Geometry check sheet. Reference: drawing and pictorial views, mm from the part's lowest x, y, z. A direction names the side the tool comes from. Round coordinates to 2 decimals unless told otherwise and drop trailing zeros. Order: outer loops, then holes, each group sorted by start corner. A loop starts at its lowest first (then second) coordinate and runs counter-clockwise, first axis right, second up.
(1) Set-up check for the marked faces 1, 2 and 3: record each of +Z, -Z, +X, -X, +Y, -Y from which the full face is reachable in a straight line by a thin tool's end or side.
(2) Go/stop test with flat-tipped pins: pin 1 (3 mm diameter, centred on y = 16.5, z = 2.5, fed in from +X); pin 2 (3.5 mm diameter, centred on x = 41.5, z = 7, fed in from -Y); pin 3 (3 mm diameter, centred on x = 48.5, z = 8.5, fed in from +Y). Record where each tip stops, or that it passes through.
(3) Sectioned sample at A-A (x = 54.5). Record the boundary of the cut face in (y, z).
(4) Sectioned sample at C-C (z = 7.5). Record the boundary of the cut face in (x, y).
(5) Sectioned sample at D-D (x = 38). Record the boundary of the cut face in (y, z).
(6) Sectioned sample at B-B (y = 79.5). Record the boundary of the cut face in (x, z).
(7) Release check for a two-part mould opening along X. For the marked faces 4, 5, 6 and 7 record: +X half, -X half, draft (parallel to the pull), parting line (faces both ways), or undercut.
(8) Material ranges on line 1 along X through (y, z) = (15, 3.95); line 2 along X through (y, z) = (80, 6.75); line 3 along Y through (x, z) = (102.5, 8.5), recorded low to high.
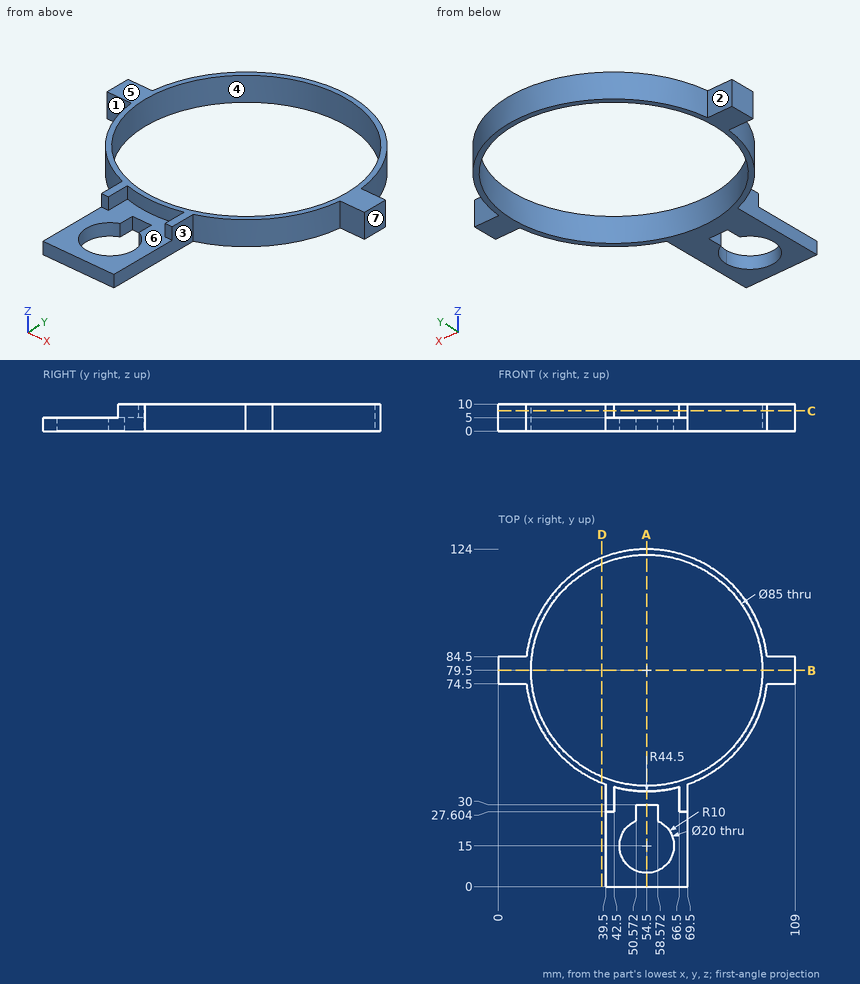
Answer below:
1. face 1: +Z, -Z, -X, -Y
1. face 2: +Z, -Z, -X, +Y
1. face 3: +Z, -Z, +X, -Y
2. pin 1: stops at x = 69.5
2. pin 2: stops at y = 27.6
2. pin 3: stops at y = 123.77
3. outline: (0, 0) - (5, 0) - (5, 5) - (0, 5) - close; (30, 0) - (37, 0) - (37, 10) - (35, 10) - (35, 5) - (30, 5) - close; (122, 0) - (124, 0) - (124, 10) - (122, 10) - close
4. outline: (0, 74.5) - (10.28, 74.5) arc R44.5 ccw to (39.5, 37.6) - (39.5, 27.6) - (42.5, 27.6) - (42.5, 36.65) arc R44.5 ccw to (66.5, 36.65) - (66.5, 27.6) - (69.5, 27.6) - (69.5, 37.6) arc R44.5 ccw to (98.72, 74.5) - (109, 74.5) - (109, 84.5) - (98.72, 84.5) arc R44.5 ccw to (10.28, 84.5) - (0, 84.5) - close; hole circle Ø85 at (54.5, 79.5)
5. outline: (38.17, 0) - (40.33, 0) - (40.33, 10) - (38.17, 10) - close; (118.67, 0) - (120.83, 0) - (120.83, 10) - (118.67, 10) - close
6. outline: (0, 0) - (12, 0) - (12, 10) - (0, 10) - close; (97, 0) - (109, 0) - (109, 10) - (97, 10) - close
7. face 4: undercut
7. face 5: draft
7. face 6: undercut
7. face 7: +X half
8. line 1: x = 39.5 to 44.5, 64.5 to 69.5
8. line 2: x = 0 to 12, 97 to 109
8. line 3: y = 74.5 to 84.5
